The figure shows three views and two pictorial views of one solid part (mm, origin at its lowest corner). Answer the questions. A direction names the side the tool comes from. Round coordinates to 2 decimals unless told otherwise and drop trailing zeros. Order: outer loops, then holes, each group sorted by start corner. A loop starts at its lowest first (then second) coordinate and runs counter-clockwise, first axis right, second up. Notation, with made-up numbers: (-7.5, -11.5) - (43.5, -11.5) arc R36 cw to (43.5, 22.5) - close; hole circle Ø2 at (-35, 47). An arc over 180 degrees is marked (long way). One line per item, written item: value. Start each with the question number.
1. Flat-ended cylindrical pins translate along their axes: P1, Ø5, axis at x = 20, z = 5, coming from the +Y side; P2, Ø2, axis at x = 7, z = 2, coming from the +Y side; P3, Ø3, axis at x = 17, z = 7.5, coming from the +Y side. Find the tip coordinate at first contact, or state that the pin passes through.
2. Straight lines are drawn through the part: line 1 (X direction, y = 0.7, z = 5); line 2 (Z direction, x = 4, y = 0.5); line 3 (X direction, y = 0.3, z = 5). For each, find the intervals that lie inside material, in ascending order.
3. A tool of negligible diameter and unlimited length cuts with its end or side. For the marked faces 1, 2 and 3, from which of +Z, -Z, +X, -X, +Y, -Y can it reach the whole face along a straight path? Write none if from no direction.
4. For a pull along X with two mould halves and no side action, classify the marked faces 4, 5 and 6 as released by +X, released by -X, zero draft, split by the parting line, or undercut.
5. Section B-B, the plane z = 5 is taken. Give the vertices of the cut face in (x, y).
6. Section A-A, the plane x = 4 is taken. Give the vertices of the cut face in (y, z).
7. Section C-C, the plane z = 2.5 is taken. Give the vertices of the cut face in (x, y).
8. Section D-D, the plane y = 3.5 is taken. Give the vertices of the cut face in (x, z), then the cut area to 3 significant figures.
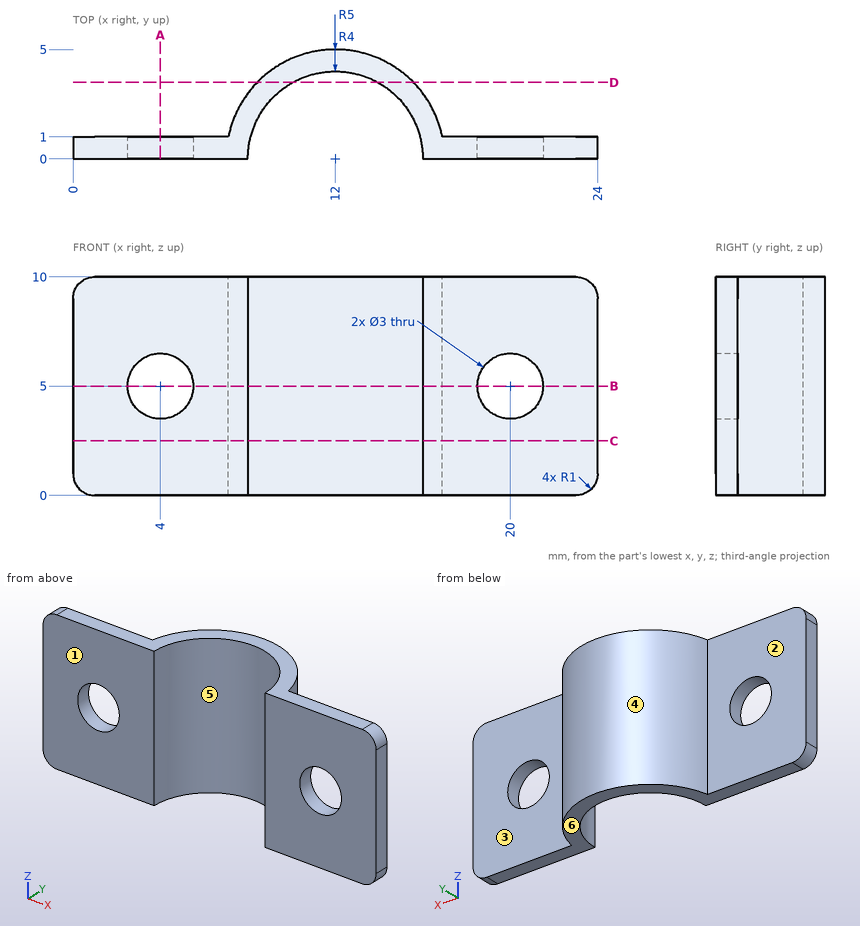
Answer list:
1. P1: stops at y = 1
1. P2: stops at y = 3
1. P3: stops at y = 3.57
2. line 1: x = 0 to 2.5, 5.5 to 8.06, 15.94 to 18.5, 21.5 to 24
2. line 2: z = 0 to 3.5, 6.5 to 10
2. line 3: x = 0 to 2.5, 5.5 to 8.01, 15.99 to 18.5, 21.5 to 24
3. face 1: +Z, -Z, +X, -X, -Y
3. face 2: +Z, -Z, -X, +Y
3. face 3: +Z, -Z, +X, +Y
4. face 4: split by the parting line
4. face 5: undercut
4. face 6: zero draft
5. outline: (0, 0) - (2.5, 0) - (2.5, 1) - (0, 1) - close; (5.5, 0) - (8, 0) arc R4 cw to (16, 0) - (18.5, 0) - (18.5, 1) - (16.9, 1) arc R5 ccw to (7.1, 1) - (5.5, 1) - close; (21.5, 0) - (24, 0) - (24, 1) - (21.5, 1) - close
6. outline: (0, 0) - (1, 0) - (1, 3.5) - (0, 3.5) - close; (0, 6.5) - (1, 6.5) - (1, 10) - (0, 10) - close
7. outline: (0, 0) - (8, 0) arc R4 cw to (16, 0) - (24, 0) - (24, 1) - (16.9, 1) arc R5 ccw to (7.1, 1) - (0, 1) - close
8. outline: (8.43, 0) - (10.06, 0) - (10.06, 10) - (8.43, 10) - close; (13.94, 0) - (15.57, 0) - (15.57, 10) - (13.94, 10) - close
8. area: 32.7 mm²
